Verification items for the finished model (mm, model axes). A direction names the side the tool comes from. Round coordinates to 2 decimals unless told otherwise and drop trailing zeros. Write each loop counter-clockwise with the first axis right and the second up, starting at its lowest first coordinate (ties: lowest second). Pieces come first, ordered by that corner, then holes. Notation, with made-up numbers: M 1.5,60.25 L 41.5,60.25 A28 cw 41.5,88.25 Z; hole C 53.25,-8.75 d11. An arc over 180 degrees is marked long. Answer in a Markdown table with one row per item. Add a question column.
1. Sectioned sample at D-D on y = -40. Record the cut outline in (x, z).
2. Set-up check for faces 1 (the cylindrical face through (24.986, 23.647, -11.521)), 2 (the flat face through (0, -25.75, -12)): record each of +Z, -Z, +X, -X, +Y, -Y from which the full face is reachable in a straight line by a thin tool's end or side.
3. Draft check along X on faces 3 (the cylindrical face through (21.21, -54.89, -11.52)), 4 (the flat face through (12.11, -57.14, -11.52)), 5 (the flat face through (0, 29.35, -12)), 6 (the cylindrical face through (31.721, -25.886, -11.521)). Enter one of: pulls with the +X half, pulls with the -X half, needs draft (parallel to the pull), parting line crosses it, or undercut.
4. Go/stop test with flat-tipped pins: pin 1 Ø1.5 at (x, z) = (6.5, -11.5) entering from -Y; pin 2 Ø0.9 at (y, z) = (-14.5, -11.5) entering from +X; pin 3 Ø1.5 at (y, z) = (24.5, -11) entering from +X. Record where each tip stops, or that it passes through.
5. Material ranges on probe 1 along Y at (x, z) = (-5, -10.85); probe 2 along X at (y, z) = (-22.5, -11.15); probe 3 along Y at (x, z) = (21, -12.2), recorded low to high.
6. Sectioned sample at B-B on y = 15. Record the cut outline in (x, z).
7. Sectioned sample at C-C on x = 21. Record the cut outline in (y, z).
8. Sectioned sample at A-A on x = -5. Record the cut outline in (y, z).
```python
from build123d import *

# Parameters (mm, degrees)
ESBO_O1_R                = 1.6
ESBO_O1_R_2              = 3
RESSALTO_EXTRUS_O1_DEPTH = 3


with BuildPart() as part:
    # Esboço1 → Ressalto-extrusão1 (new body)
    with BuildSketch(Plane(origin=(0, 0, -13), x_dir=(-1, 0, 0), z_dir=(0, 0, -1))):
        with BuildLine():
            Line((11, 29.35), (-11, 29.35))
            ThreePointArc((-11, 29.35), (-25.142135624, 23.492135624), (-31, 9.35))
            Line((-31, 9.35), (-31, -23.298998166))
            ThreePointArc((-31, -23.298998166), (-31.741318167, -25.918851033), (-33.745451618, -27.76184609))
            Line((-33.745451618, -27.76184609), (-36.710953382, -29.259962834))
            ThreePointArc((-36.710953382, -29.259962834), (-38.715086833, -31.102957891), (-39.456405, -33.722810758))
            Line((-39.456405, -33.722810758), (-39.456405, -49.230667326))
            ThreePointArc((-39.456405, -49.230667326), (-38.715086833, -51.850520194), (-36.710953382, -53.693515251))
            Line((-36.710953382, -53.693515251), (-23.254548382, -60.491442635))
            ThreePointArc((-23.254548382, -60.491442635), (-21, -61.028594711), (-18.745451618, -60.491442635))
            Line((-18.745451618, -60.491442635), (-5.289046618, -53.693515251))
            ThreePointArc((-5.289046618, -53.693515251), (-3.284913167, -51.850520194), (-2.543595, -49.230667326))
            Line((-2.543595, -49.230667326), (-2.543595, -35.646914307))
            ThreePointArc((-2.543595, -35.646914307), (-1.079128906, -32.111380402), (2.456405, -30.646914307))
            Line((2.456405, -30.646914307), (11, -30.646914307))
            ThreePointArc((11, -30.646914307), (14.535533906, -29.182448213), (16, -25.646914307))
            Line((16, -25.646914307), (16, 24.35))
            ThreePointArc((16, 24.35), (14.535533906, 27.885533906), (11, 29.35))
        make_face()
        with Locations((-5, -24.75)):
            Circle(ESBO_O1_R, mode=Mode.SUBTRACT)
        with Locations((-5, 24.75)):
            Circle(ESBO_O1_R, mode=Mode.SUBTRACT)
        with Locations((5, -24.75)):
            Circle(ESBO_O1_R, mode=Mode.SUBTRACT)
        with Locations((5, 24.75)):
            Circle(ESBO_O1_R, mode=Mode.SUBTRACT)
        with Locations((-21, 15)):
            Circle(ESBO_O1_R, mode=Mode.SUBTRACT)
        with Locations((-21, -15)):
            Circle(ESBO_O1_R, mode=Mode.SUBTRACT)
        with Locations((-7.143595, -33.476739042)):
            Circle(ESBO_O1_R, mode=Mode.SUBTRACT)
        with Locations((-7.143595, -49.476739042)):
            Circle(ESBO_O1_R, mode=Mode.SUBTRACT)
        with Locations((-21, -26.476739042)):
            Circle(ESBO_O1_R, mode=Mode.SUBTRACT)
        with Locations((-21, -56.476739042)):
            Circle(ESBO_O1_R, mode=Mode.SUBTRACT)
        with Locations((-21, -41.476739042)):
            Circle(ESBO_O1_R_2, mode=Mode.SUBTRACT)
        with Locations((-34.856405, -33.476739042)):
            Circle(ESBO_O1_R, mode=Mode.SUBTRACT)
        with Locations((-34.856405, -49.476739042)):
            Circle(ESBO_O1_R, mode=Mode.SUBTRACT)
        Polygon((-1.5, -21), (-11, -21), (-11, 21), (-1.5, 21), (-1.5, 25.75), (1.5, 25.75), (1.5, 21), (11, 21), (11, -21), (1.5, -21), (1.5, -25.75), (-1.5, -25.75), align=None, mode=Mode.SUBTRACT)
    extrude(amount=-RESSALTO_EXTRUS_O1_DEPTH)


solid = part.part
```
Geometry check:
| question | item | result |
|---|---|---|
| 1 | outline | M 2.54,-13 L 18.39,-13 L 18.39,-10 L 2.54,-10 Z; M 23.61,-13 L 39.46,-13 L 39.46,-10 L 23.61,-10 Z |
| 2 | face 1 | +Z, -Z, +X, +Y |
| 2 | face 2 | +Z, -Z |
| 3 | face 3 | undercut |
| 3 | face 4 | pulls with the -X half |
| 3 | face 5 | needs draft |
| 3 | face 6 | pulls with the +X half |
| 4 | pin 1 | stops at y = -54.68 |
| 4 | pin 2 | stops at x = 31 |
| 4 | pin 3 | stops at x = 24.88 |
| 5 | probe 1 | y = -30.65 to -26.35, -23.15 to -21, 21 to 23.15, 26.35 to 29.35 |
| 5 | probe 2 | x = -16 to -1.5, 1.5 to 31 |
| 5 | probe 3 | y = -61.03 to -58.08, -54.88 to -44.48, -38.48 to -28.08, -24.88 to -16.6, -13.4 to 13.4, 16.6 to 26.67 |
| 6 | outline | M -16,-13 L -11,-13 L -11,-10 L -16,-10 Z; M 11,-13 L 19.4,-13 L 19.4,-10 L 11,-10 Z; M 22.6,-13 L 30.19,-13 L 30.19,-10 L 22.6,-10 Z |
| 7 | outline | M -61.03,-13 L -58.08,-13 L -58.08,-10 L -61.03,-10 Z; M -54.88,-13 L -44.48,-13 L -44.48,-10 L -54.88,-10 Z; M -38.48,-13 L -28.08,-13 L -28.08,-10 L -38.48,-10 Z; M -24.88,-13 L -16.6,-13 L -16.6,-10 L -24.88,-10 Z; M -13.4,-13 L 13.4,-13 L 13.4,-10 L -13.4,-10 Z; M 16.6,-13 L 26.67,-13 L 26.67,-10 L 16.6,-10 Z |
| 8 | outline | M -30.65,-13 L -26.35,-13 L -26.35,-10 L -30.65,-10 Z; M -23.15,-13 L -21,-13 L -21,-10 L -23.15,-10 Z; M 21,-13 L 23.15,-13 L 23.15,-10 L 21,-10 Z; M 26.35,-13 L 29.35,-13 L 29.35,-10 L 26.35,-10 Z |
